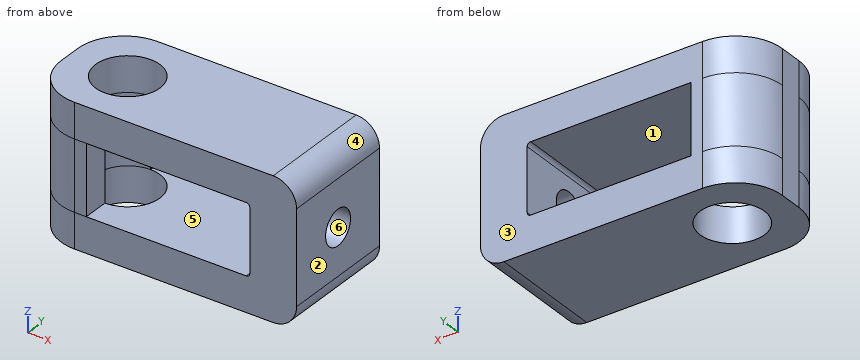
from build123d import *
from build123d.topology import SkipClean

# Parameters (mm, degrees)
EXTRUDE_1_DEPTH     = 10
SKETCH_2_R          = 2.75
CUT_EXTRUDE_1_DEPTH = 16
FILLET_1_R          = 4
SKETCH_3_R          = 1.5
CUT_EXTRUDE_2_DEPTH = 10
FILLET_2_R          = 2
FILLET_3_R          = 0.3
EXTRUDE_4_DEPTH     = 6


with BuildPart() as part:
    # 草图1 → 凸台-拉伸1 (new body)
    with BuildSketch(Plane(origin=(0, 0, 0), x_dir=(1, 0, 0), z_dir=(0, 1, 0))):
        Polygon((0, 3), (-19, 3), (-19, 6), (0, 6), (4, 6), (4, -6), (0, -6), (-19, -6), (-19, -3), (0, -3), align=None)
    extrude(amount=EXTRUDE_1_DEPTH)

    # 草图2 → 切除-拉伸1 (cut)
    with BuildSketch(Plane.XY.offset(6)):
        with Locations((-14, 5)):
            Circle(SKETCH_2_R)
    extrude(amount=-CUT_EXTRUDE_1_DEPTH, mode=Mode.SUBTRACT)

    # 圆角1
    fillet_1_edges = [part.edges().sort_by_distance(p)[0] for p in [
        (-19, 0, -4.5),
        (-19, 10, 4.5),
        (-19, 0, 4.5),
        (-19, 10, -4.5),
    ]]
    fillet(fillet_1_edges, radius=FILLET_1_R)

    # 草图3 → 切除-拉伸2 (cut)
    with BuildSketch(Plane(origin=(4, 0, 0), x_dir=(0, 0, -1), z_dir=(1, 0, 0))):
        with Locations((0, 5)):
            Circle(SKETCH_3_R)
    extrude(amount=-CUT_EXTRUDE_2_DEPTH, mode=Mode.SUBTRACT)

    # 圆角2
    fillet_2_edges = [part.edges().sort_by_distance(p)[0] for p in [
        (4, 5, -6),
        (4, 5, 6),
    ]]
    fillet(fillet_2_edges, radius=FILLET_2_R)

    # 圆角3
    fillet_3_edges = [part.edges().sort_by_distance(p)[0] for p in [
        (0, 5, -3),
        (0, 5, 3),
    ]]
    fillet(fillet_3_edges, radius=FILLET_3_R)

    # 草图9 → 凸台-拉伸4 (add)
    with SkipClean():  # the faces are left unmerged after this step: merging them gives an invalid solid
        with BuildSketch(Plane.XY.offset(-3)):
            with BuildLine():
                ThreePointArc((-15, 10), (-17.828427125, 8.828427125), (-19, 6))
                Line((-19, 6), (-19, 4))
                ThreePointArc((-19, 4), (-17.828427125, 1.171572875), (-15, 0))
                Line((-15, 0), (-14, 0))
                Line((-14, 0), (-14, 2.25))
                ThreePointArc((-14, 2.25), (-16.75, 5), (-14, 7.75))
                Line((-14, 7.75), (-14, 10))
                Line((-14, 10), (-15, 10))
            make_face()
        extrude(amount=EXTRUDE_4_DEPTH)


solid = part.part
The model under review builds one solid part; all positions refer to its coordinate system, in mm. Face numbers are marked on the shaded views. A direction names the side the tool comes from. Round coordinates to 2 decimals unless told otherwise and drop trailing zeros. Order: outer loops, then holes, each group sorted by start corner. A loop starts at its lowest first (then second) coordinate and runs counter-clockwise, first axis right, second up. Notation, with made-up numbers: (-34.5, 56) -> (24.5, 56) arc R23 cw to (24.5, 79) -> close; hole circle Ø11 at (2.5, 17.5). An arc over 180 degrees is marked (long way). Return JSON: item names as keys, results as strings.
1. The part is to be moulded in two halves that separate along X. For the marked faces 1, 2 and 3, say which applies: +X half, -X half, draft (parallel to the pull), parting line (faces both ways), or undercut.
Answer block:
{"face 1": "undercut", "face 2": "+X half", "face 3": "draft"}
2. Take a section at B-B (z = 0). Write out the cut boundary in (x, y), then the cut area to 3 significant figures.
Answer block:
{"outline": "(-19, 4) arc R4 ccw to (-15, 0) -> (-14, 0) -> (-14, 2.25) arc R2.75 cw to (-14, 7.75) -> (-14, 10) -> (-15, 10) arc R4 ccw to (-19, 6) -> close; (0, 0) -> (4, 0) -> (4, 3.5) -> (0, 3.5) -> close; (0, 6.5) -> (4, 6.5) -> (4, 10) -> (0, 10) -> close", "area": "59.3 mm²"}
3. Take a section at C-C (y = 5). Write out the cut boundary in (x, z), then the cut area to 3 significant figures.
Answer block:
{"outline": "(-19, -6) -> (-16.75, -6) -> (-16.75, 6) -> (-19, 6) -> close; (-11.25, -6) -> (2, -6) arc R2 ccw to (4, -4) -> (4, -1.5) -> (0, -1.5) -> (0, -2.7) arc R0.3 cw to (-0.3, -3) -> (-11.25, -3) -> close; (-11.25, 3) -> (-0.3, 3) arc R0.3 cw to (0, 2.7) -> (0, 1.5) -> (4, 1.5) -> (4, 4) arc R2 ccw to (2, 6) -> (-11.25, 6) -> close", "area": "129 mm²"}
4. For the marked faces 4, 5 and 6, list the 3-axis set-ups (+Z, -Z, +X, -X, +Y, -Y) from which the entire face can be reached by the end or side of a thin tool; tool diameter is ignored.
Answer block:
{"face 4": "+Z, +X, +Y, -Y", "face 5": "+Y, -Y", "face 6": "+X"}
5. Insertion check: P1, Ø1.5, axis at x = -2, z = 1, coming from the +Y side. The pin has a flat end and moves straight along its axis. Give the tip position at first contact, or say it passes through.
Answer block:
{"P1": "passes through"}
6. Take a section at D-D (x = -3.5). Write out the cut boundary in (y, z).
Answer block:
{"outline": "(0, -6) -> (10, -6) -> (10, -3) -> (0, -3) -> close; (0, 3) -> (10, 3) -> (10, 6) -> (0, 6) -> close"}
7. For L1, parallel to Z at x = -4.5, y = 6.25; L2, parallel to X at y = 5, z = 4; L3, parallel to Y at x = -14, z = -5.1, list the stretches that pass through material, from the lowest coordinate up. Write a range as [from, to].
Answer block:
{"L1": "z = [-6, -3], [3, 6]", "L2": "x = [-19, -16.75], [-11.25, 4]", "L3": "y = [0, 2.25], [7.75, 10]"}
8. Take a section at A-A (z = 1.75). Write out the cut boundary in (x, y), then the cut area to 3 significant figures.
Answer block:
{"outline": "(-19, 4) arc R4 ccw to (-15, 0) -> (-14, 0) -> (-14, 2.25) arc R2.75 cw to (-14, 7.75) -> (-14, 10) -> (-15, 10) arc R4 ccw to (-19, 6) -> close; (0, 0) -> (4, 0) -> (4, 10) -> (0, 10) -> close", "area": "71.3 mm²"}
